Build history of the part. All positions in model axes, mm. A direction names the side the tool comes from. Round coordinates to 2 decimals unless told otherwise and drop trailing zeros. Write each loop counter-clockwise with the first axis right and the second up, starting at its lowest first coordinate (ties: lowest second). Pieces come first, ordered by that corner, then holes. Notation, with made-up numbers: M 7.25,-21 L 45.25,-21 A25 cw 45.25,-9 Z; hole C -27.5,-11.5 d11. An arc over 180 degrees is marked long. Write item = value, one per line. Start each with the question number.
Q1. Band-saw the part on D-D on z = 0.9. Write the cut outline in (x, y) (3 decimals).
Q2. Band-saw the part on B-B on x = 0. Write the cut outline in (y, z) (3 decimals).
Q3. Band-saw the part on C-C on y = 5.25. Write the cut outline in (x, z).
Q4. Probe L1, parallel to Y at x = -0.25, z = -1.1; L2, parallel to Y at x = 2, z = -0.2; L3, parallel to X at y = 6.25, z = -0.15. List the from-to ranges inside material, lowest first.
Q5. Tool access for faces 1 (the flat face through (0, 2, 1.524)), 2 (the flat face through (-1.524, 2, 0)), 3 (the flat face through (0, 2, -1.524)), 4 (the flat face through (3, 9.55, 0)), 5 (the flat face through (4.5, 12.7, -1.3)): list every direction of +Z, -Z, +X, -X, +Y, -Y with a clear straight run to the whole face (end or side of a thin tool).
Q6. Band-saw the part on A-A on z = -0.6. Write the cut outline in (x, y) (3 decimals).
Q7. Drop flat-ended pins along their axis: P1, Ø0.9, axis at x = 0.5, y = 1.5, coming from the +Z side; P2, Ø0.9, axis at x = 0, y = 1, coming from the -Z side; P3, Ø0.9, axis at y = 1.5, z = 0, coming from the +X side. Give the stop position or say it passes through.
Autodesk Inventor part; units mm, degrees
ref_plane "YZ Plane" through (0, 0, 0) normal (1, 0, 0) x (0, 1, 0)
ref_plane "XZ Plane" through (0, 0, 0) normal (0, 1, 0) x (-1, 0, 0)
ref_plane "XY Plane" through (0, 0, 0) normal (0, 0, 1) x (1, 0, 0)
sketch "Sketch1" plane through (0, 0, 0) normal (0, 1, 0) x (-1, 0, 0)
  line L0 (-1.5748, 1.5748) -> (1.5748, 1.5748)
  line L1 (1.5748, 1.5748) -> (1.5748, -1.5748)
  line L2 (1.5748, -1.5748) -> (-1.5748, -1.5748)
  line L3 (-1.5748, -1.5748) -> (-1.5748, 1.5748)
  line L4 (-1.5748, 1.5748) -> (1.5748, -1.5748) construction
  line L5 (1.5748, 1.5748) -> (-1.5748, -1.5748) construction
  point P0 (0, 0)
  dimension "d0" = 3.1496
  dimension "d1" = 3.1496
extrude "Extrusion1" add sketch "Sketch1" along normal blind 6.35
sketch "Sketch2" plane through (-1.5748, 0, 1.5748) normal (0, 0, 1) x (1, 0, 0)
  line L0 (3.1496, 0) -> (0, 0)
  line L1 (3.1496, 0) -> (0, 0)
  line L2 (0, 0) -> (0, 12.7)
  line L3 (0, 12.7) -> (3.1496, 12.7)
  line L4 (3.1496, 12.7) -> (3.1496, 0)
  line L5 (0, 12.7) -> (6.35, 12.7)
  line L6 (6.35, 12.7) -> (6.35, 9.5504)
  line L7 (6.35, 9.5504) -> (0, 9.5504)
  line L8 (0, 9.5504) -> (0, 12.7)
  point P0 (1.5748, 0)
  point P1 (3.1496, 9.5504)
  dimension "d4" = 12.7
  dimension "d5" = 6.35
  dimension "d6" = 3.1496
extrude "Extrusion2" add sketch "Sketch2" against normal blind 3.1496
sketch "Sketch3" plane through (-1.5748, 12.7, 1.5748) normal (0, 1, 0) x (1, 0, 0)
  line L0 (0, 3.1496) -> (6.35, 3.1496)
  line L1 (6.35, 3.1496) -> (3.2004, 3.1496)
  line L2 (3.2004, 3.1496) -> (3.2004, 0)
  line L3 (3.2004, 0) -> (6.35, 0)
  line L4 (6.35, 0) -> (6.35, 3.1496)
  circle A0 centre (4.7752, 1.5748) radius 1.5748
  point P0 (1.5748, 1.5748)
  dimension "d9" = 3.1496
  dimension "d10" = 3.1496
extrude "Extrusion3" add sketch "Sketch3" along normal blind 6.35 contours A0
sketch "Sketch4" plane through (0, 0, 0) normal (0, -1, 0) x (1, 0, 0)
  line L0 (1.5748, -1.5748) -> (-1.5748, -1.5748)
  line L1 (1.5748, 1.5748) -> (1.5748, -1.5748)
  line L2 (1.6002, 1.5748) -> (-1.5748, 1.5748)
  line L3 (-1.5748, -1.5748) -> (-1.5748, 1.5748)
  line L4 (1.524, 1.524) -> (-1.524, 1.524)
  line L5 (-1.524, 1.524) -> (-1.524, -1.524)
  line L6 (-1.524, -1.524) -> (1.524, -1.524)
  line L7 (1.524, -1.524) -> (1.524, 1.524)
  line L8 (1.524, 1.524) -> (-1.524, -1.524) construction
  line L9 (-1.524, 1.524) -> (1.524, -1.524) construction
  point P0 (0, 0)
  dimension "d13" = 3.048
  dimension "d14" = 3.048
extrude "Extrusion4" cut sketch "Sketch4" against normal blind 3.175
properties part number "Handle"
Conclusion:
q1.outline = M -1.575,3.175 L -1.524,3.175 L -1.524,0 L 1.524,0 L 1.524,3.175 L 1.575,3.175 L 1.575,9.55 L 4.775,9.55 L 4.775,12.7 L 4.493,12.7 L 4.493,19.05 L 1.908,19.05 L 1.908,12.7 L -1.575,12.7 Z
q2.outline = M 0,-1.524 L 3.175,-1.524 L 3.175,-1.575 L 12.7,-1.575 L 12.7,1.575 L 3.175,1.575 L 3.175,1.524 L 0,1.524 Z
q3.outline = M -1.57,-1.57 L 1.57,-1.57 L 1.57,1.57 L -1.57,1.57 Z
q4.L1 = 0 to 12.7
q4.L2 = 9.55 to 19.05
q4.L3 = -1.57 to 1.57
q5.face_1 = +Z, +X, -X, -Y
q5.face_2 = +Z, -Z, -X, -Y
q5.face_3 = -Z, +X, -X, -Y
q5.face_4 = +Z, -Z, +X, -Y
q5.face_5 = -Z, +X, +Y
q6.outline = M -1.575,3.175 L -1.524,3.175 L -1.524,0 L 1.524,0 L 1.524,3.175 L 1.575,3.175 L 1.575,9.55 L 4.775,9.55 L 4.775,12.7 L 4.656,12.7 L 4.656,19.05 L 1.744,19.05 L 1.744,12.7 L -1.575,12.7 Z
q7.P1 = 1.52
q7.P2 = -1.52
q7.P3 = 1.52
